Geometry: final body of the model. Coordinates: model frame, mm. Coordinates: 2 decimals unless noted, no trailing zeros. Write each loop counter-clockwise with the first axis right and the second up, starting at its lowest first coordinate (ties: lowest second). Pieces come first, ordered by that corner, then holes. Notation, with made-up numbers: (-12.75, -25.5) -> (4.25, -25.5) arc R15 cw to (4.25, -8.5) -> close; hole circle Ø9 at (89, -16.75). An arc over 180 degrees is marked (long way). One line per item, written item: value.
```python
from build123d import *

# Parameters (mm, degrees)
BOSS_EXTRUDE1_DEPTH = 0.254
SKETCH2_R           = 4.699
CUT_EXTRUDE1_DEPTH  = 1.254
SKETCH3_W           = 2.54
SKETCH3_H           = 0.635
CUT_EXTRUDE2_DEPTH  = 1.254
SKETCH5_OUTSIDE_W   = 121.447
SKETCH5_OUTSIDE_H   = 109.618
SKETCH5_OUTSIDE_W_2 = 14.224
SKETCH5_OUTSIDE_H_2 = 15.24
CUT_EXTRUDE5_DEPTH  = 1.254


with BuildPart() as part:
    # Sketch1 → Boss-Extrude1 (new body)
    with BuildSketch(Plane.XY):
        with BuildLine():
            Line((67.21146711, 76.191723231), (8.696654013, 17.676910134))
            Line((8.696654013, 17.676910134), (7.228954972, 14.133571205))
            ThreePointArc((7.228954972, 14.133571205), (14.666587579, 6.075099489), (15.105587123, -4.88230096))
            Line((15.105587123, -4.88230096), (18.648926052, -6.35))
            Line((18.648926052, -6.35), (101.401368334, -6.35))
            ThreePointArc((101.401368334, -6.35), (93.866160503, 38.880636728), (67.21146711, 76.191723231))
        make_face()
        with BuildLine():
            Line((88.672924278, 6.35), (27.86051193, 6.35))
            ThreePointArc((27.86051193, 6.35), (26.399857642, 10.93517908), (24.190484974, 15.210228852))
            Line((24.190484974, 15.210228852), (67.191354125, 58.211098004))
            ThreePointArc((67.191354125, 58.211098004), (82.13289044, 34.020557137), (88.672924278, 6.35))
        make_face(mode=Mode.SUBTRACT)
    extrude(amount=BOSS_EXTRUDE1_DEPTH)

    # Sketch2 → Cut-Extrude1 (cut, through all)
    with BuildSketch(Plane.XY.offset(0.254)):
        with Locations((22.225, 0)):
            Circle(SKETCH2_R)
        with Locations((36.195, 0)):
            Circle(SKETCH2_R)
        with Locations((61.722, 0)):
            Circle(SKETCH2_R)
        with Locations((75.692, 0)):
            Circle(SKETCH2_R)
        with Locations((95.25, 0)):
            Circle(SKETCH2_R)
        with Locations((15.715448212, 15.715448212)):
            Circle(SKETCH2_R)
        with Locations((25.593729945, 25.593729945)):
            Circle(SKETCH2_R)
        with Locations((43.644044748, 43.644044748)):
            Circle(SKETCH2_R)
        with Locations((53.522326482, 53.522326482)):
            Circle(SKETCH2_R)
        with Locations((92.004434954, 24.652514046)):
            Circle(SKETCH2_R)
        with Locations((82.48891971, 47.625)):
            Circle(SKETCH2_R)
        with Locations((67.351920908, 67.351920908)):
            Circle(SKETCH2_R)
    extrude(amount=-CUT_EXTRUDE1_DEPTH, mode=Mode.SUBTRACT)

    # Sketch3 → Cut-Extrude2 (cut, through all)
    with BuildSketch(Plane.XY.offset(0.254)):
        Polygon((15.266435406, 24.246691527), (17.06248663, 26.042742751), (17.511499436, 25.593729945), (15.715448212, 23.797678721), align=None)
        Polygon((44.991083167, 53.971339288), (43.195031942, 52.175288063), (43.644044748, 51.726275257), (45.440095973, 53.522326482), align=None)
        with Locations((29.21, -6.0325)):
            Rectangle(SKETCH3_W, SKETCH3_H)
        with Locations((68.707, -6.0325)):
            Rectangle(SKETCH3_W, SKETCH3_H)
        Polygon((29.230733674, 38.210989795), (31.026784898, 40.007041019), (31.475797704, 39.558028213), (29.67974648, 37.761976989), align=None)
        Polygon((56.845021246, 65.825277367), (55.048970022, 64.029226143), (55.497982828, 63.580213337), (57.294034052, 65.376264561), align=None)
        with Locations((48.9585, -6.0325)):
            Rectangle(SKETCH3_W, SKETCH3_H)
        with Locations((85.471, -6.0325)):
            Rectangle(SKETCH3_W, SKETCH3_H)
        Polygon((99.935462164, 14.437711971), (100.266998693, 11.919442024), (101.526133667, 12.085210288), (101.194597138, 14.603480236), align=None)
        Polygon((93.765504959, 37.464305742), (94.938831965, 37.950313702), (93.966816047, 40.296967714), (92.793489041, 39.810959755), align=None)
        Polygon((79.327792988, 62.471156422), (80.874047017, 60.456038938), (81.88160576, 61.229165953), (80.33535173, 63.244283437), align=None)
        Polygon((13.593916116, 7.005422516), (14.565932035, 4.658768503), (15.739259041, 5.144776462), (14.767243123, 7.491430475), align=None)
    extrude(amount=-CUT_EXTRUDE2_DEPTH, mode=Mode.SUBTRACT)

    # Sketch5 outside → Cut-Extrude5 (cut, through all)
    with BuildSketch(Plane.XY.offset(0.254)):
        with Locations((54.4145, 34.921)):
            Rectangle(SKETCH5_OUTSIDE_W, SKETCH5_OUTSIDE_H)
        with Locations((77.089, 0)):
            Rectangle(SKETCH5_OUTSIDE_W_2, SKETCH5_OUTSIDE_H_2, mode=Mode.SUBTRACT)
    extrude(amount=-CUT_EXTRUDE5_DEPTH, mode=Mode.SUBTRACT)


solid = part.part
```
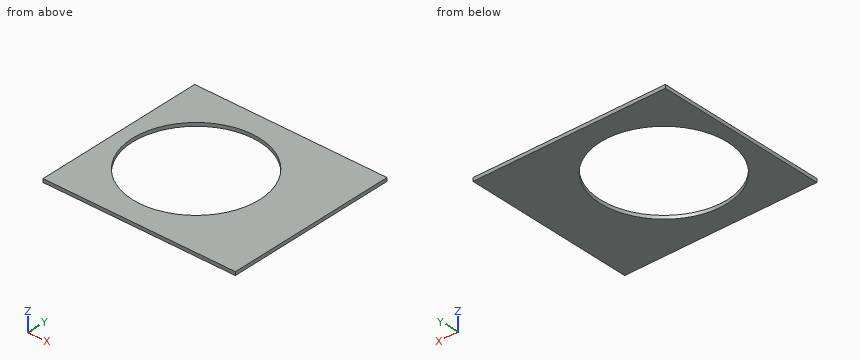
(1) Line query: line 1 (Y direction, x = 75.5, z = 0.2); line 2 (Y direction, x = 78.5, z = 0.2); line 3 (X direction, y = 3.25, z = 0.05). Output: solid intervals per line, ascending. Write a range as [from, to].
Responses:
line 1: y = [-6.35, -4.7], [4.7, 6.35]
line 2: y = [-6.35, -3.77], [3.77, 6.35]
line 3: x = [69.98, 72.3], [79.09, 84.2]
(2) First-contact query: pin 1 (5.5 mm diameter, centred on x = 75.692, y = 0, fed in from -Z). Flat tip, straight axial feed; report the tip coordinate or a pass-through.
Responses:
pin 1: passes through
(3) Section C-C (z = 0.15). Return the cut outline in (x, y), then the cut area to 3 significant figures.
Responses:
outline: (69.98, -6.35) -> (84.2, -6.35) -> (84.2, 6.35) -> (69.98, 6.35) -> close; hole circle Ø9.4 at (75.69, 0)
area: 111 mm2
(4) Section B-B (x = 78.25). Return the cut outline in (y, z).
Responses:
outline: (-6.35, 0) -> (-3.94, 0) -> (-3.94, 0.25) -> (-6.35, 0.25) -> close; (3.94, 0) -> (6.35, 0) -> (6.35, 0.25) -> (3.94, 0.25) -> close
(5) Section A-A (y = 0). Return the cut outline in (x, z).
Responses:
outline: (69.98, 0) -> (70.99, 0) -> (70.99, 0.25) -> (69.98, 0.25) -> close; (80.39, 0) -> (84.2, 0) -> (84.2, 0.25) -> (80.39, 0.25) -> close
